Source: CAD feature listing. Evaluate the final solid. Frame: model axes, mm. A direction names the side the tool comes from. Give positions to 0.01 mm unless a question says otherwise; leave off trailing zeros. Order: outer loops, then holes, each group sorted by start corner. A loop starts at its lowest first (then second) coordinate and runs counter-clockwise, first axis right, second up. Notation, with made-up numbers: M 51.5,52 L 89.5,52 A6 cw 89.5,62 Z; hole C 86.5,32 d11. An arc over 180 degrees is marked long. Answer as a JSON object with one key per item and string values. Group by question number.
1. Section query B-B (x = 28). Output: boundary loops of the cut face in (y, z), plus the area to 3 significant figures.
2. Pin query (flat end, axial travel): P1, Ø4, axis at y = -2, z = 5, coming from the +X side; P2, Ø4, axis at x = -56, y = 3.5, coming from the +Z side; P3, Ø12, axis at x = 25, z = 21, coming from the -Y side. Return the tip coordinate at first contact, or that it passes through.
3. Section query A-A (z = 21). Output: boundary loops of the cut face in (x, y).
4. Set-up query: faces 1 (the cylindrical face through (-58.2, 0.1, 12.5)), 2 (the flat face through (0, 0, 0)), 3 (the cylindrical face through (56.7, 0.1, 12.5)). Return all of +Z, -Z, +X, -X, +Y, -Y with unobstructed straight access to the full face (end or side cutting, diameter ignored); none if empty.
5. Material intervals for L1, parallel to X at y = 0.5, z = 3; L2, parallel to Z at x = -96, y = -0.25; L3, parallel to X at y = -1, z = 44.5, sorted ascending. Write a range as [from, to].
from build123d import *

# Parameters (mm, degrees)
SKETCH1_R                = 5
BOSS_EXTRUDE1_DEPTH      = 50
BOSS_EXTRUDE2_DEPTH      = 110
BOSS_EXTRUDE2_DEPTH_BACK = 110
SKETCH2_R                = 2.5
FILLET1_R                = 1


with BuildPart() as part:
    # Sketch1 → Boss-Extrude1 (new body)
    with BuildSketch(Plane.XY):
        Circle(SKETCH1_R)
    extrude(amount=BOSS_EXTRUDE1_DEPTH)

    # Sketch2 → Boss-Extrude2 (add, two sides: drawn at the far end of the back side and taken through both)
    with BuildSketch(Plane(origin=(0, 0, 0), x_dir=(0, 0, -1), z_dir=(1, 0, 0)).offset(-BOSS_EXTRUDE2_DEPTH_BACK)):
        with Locations((-10, 0)):
            Circle(SKETCH2_R)
    extrude(amount=BOSS_EXTRUDE2_DEPTH + BOSS_EXTRUDE2_DEPTH_BACK)

    # Fillet1
    fillet1_edges = [part.edges().sort_by_distance(p)[0] for p in [
        (-4.999960513, -0.019871133, 12.499921026),
        (4.330127047, 2.499999952, 10.000491239),
    ]]
    fillet(fillet1_edges, radius=FILLET1_R - 0.0001)  # a hair under: the kernel refuses the full size


solid = part.part
Answer sheet:
{
 "1": {"outline": "C 0,10 d5", "area": "19.6 mm^2"},
 "2": {"P1": "x = 5", "P2": "z = 12", "P3": "through"},
 "3": {"outline": "C 0,0 d10"},
 "4": {"face 1": "-X", "face 2": "-Z, +X, -X, +Y, -Y", "face 3": "+X"},
 "5": {"L1": "[-4.97, 4.97]", "L2": "[7.51, 12.49]", "L3": "[-4.9, 4.9]"}
}
